Here's how the part is built. I have some questions about the finished solid (model axes, mm). A direction names the side the tool comes from. Round coordinates to 2 decimals unless told otherwise and drop trailing zeros. Order: outer loops, then holes, each group sorted by start corner. A loop starts at its lowest first (then second) coordinate and runs counter-clockwise, first axis right, second up. Notation, with made-up numbers: (26, 60.25) -> (57, 60.25) arc R14 ccw to (57, 67.25) -> close; hole circle Ø10 at (53, 67.25). An arc over 180 degrees is marked (long way). One line per item, written item: value.
```python
from build123d import *

# Parameters (mm, degrees)
F1_DEPTH = 15
F2_R     = 1.99999
F3_R     = 2
F4_R     = 1
F5_SIZE  = 1


# Not quite as in the source:
# - a fillet or chamfer is up to 0.001 mm smaller than in the source, because OpenCascade refuses the exact size


with BuildPart() as f1:
    # F0 (on Top) → F1 (new body)
    with BuildSketch(Plane.XY):
        with BuildLine():
            Line((2.5, -29.8956518578), (0, 0))
            Line((0, 0), (27, 0))
            Line((27, 0), (27, -30))
            ThreePointArc((27, -30), (45.6594117082, -45.2970585408), (57, -24))
            Line((57, -24), (52.5277389168, -24))
            ThreePointArc((52.5277389168, -24), (45.7143401039, -41.1741167757), (31, -30))
            Line((31, -30), (31, 4))
            Line((31, 4), (-4.348458452, 4))
            Line((-4.348458452, 4), (-1.4860869144, -30.2289851911))
            Line((-1.4860869144, -30.2289851911), (2.5, -29.8956518578))
        make_face()
    extrude(amount=F1_DEPTH)

    # F2 (radius 2 in the source; OpenCascade refuses exactly that, so slightly less here)
    f2_edges = [f1.edges().sort_by_distance(p)[0] for p in [
        (2.5, -29.895652, 7.5),
        (-1.486087, -30.228985, 7.5),
        (52.527739, -24, 7.5),
        (57, -24, 7.5),
    ]]
    fillet(f2_edges, radius=F2_R)

    # F3
    f3_edges = [f1.edges().sort_by_distance(p)[0] for p in [
        (31, 4, 7.5),
        (-4.348458, 4, 7.5),
    ]]
    fillet(f3_edges, radius=F3_R)

    # F4
    f4_edges = [f1.edges().sort_by_distance(p)[0] for p in [
        (0, 0, 7.5),
        (27, 0, 7.5),
    ]]
    fillet(f4_edges, radius=F4_R)

    # F5
    f5_edges = [f1.edges().sort_by_distance(p)[0] for p in [
        (1.211964, -14.492976, 15),
        (0.351135, -0.322997, 15),
        (1.867439, -29.360721, 15),
        (13.543557, 0, 15),
        (0.506957, -30.062319, 15),
        (26.707107, -0.292893, 15),
        (-0.951156, -29.596424, 15),
        (27, -15.5, 15),
        (-2.910013, -13.201309, 15),
        (44.919918, -45.426535, 15),
        (-3.646189, 3.354006, 15),
        (56.78664, -24.391198, 15),
        (13.412885, 4, 15),
        (55.598458, -24, 15),
        (30.414214, 3.414214, 15),
        (53.989656, -24.81182, 15),
        (31, -14, 15),
        (44.32507, -41.471013, 15),
        (1.211964, -14.492976, 0),
        (0.351135, -0.322997, 0),
        (1.867439, -29.360721, 0),
        (13.543557, 0, 0),
        (0.506957, -30.062319, 0),
        (26.707107, -0.292893, 0),
        (-0.951156, -29.596424, 0),
        (27, -15.5, 0),
        (-2.910013, -13.201309, 0),
        (44.919918, -45.426535, 0),
        (-3.646189, 3.354006, 0),
        (56.78664, -24.391198, 0),
        (13.412885, 4, 0),
        (55.598458, -24, 0),
        (30.414214, 3.414214, 0),
        (53.989656, -24.81182, 0),
        (31, -14, 0),
        (44.32507, -41.471013, 0),
    ]]
    chamfer(f5_edges, length=F5_SIZE)


solid = f1.part
```
Q1. For P1, Ø3, axis at x = 51, y = -27.5, coming from the -Z side; P2, Ø6.5, axis at y = -14.5, z = 6.5, coming from the +X side; P3, Ø3, axis at y = -15.5, z = 4, coming from the -X side; P4, Ø4, axis at x = 12.5, z = 8.5, coming from the -Y side, each with a flat end and sliding along its axis, tell me the tip position at first contact or that it passes through.
Answers:
P1: through
P2: x = 31
P3: x = -2.84
P4: y = 0
Q2. Which directions (+Z, -Z, +X, -X, +Y, -Y) give clear straight access to the entire face, cutting with the end or side of a thin tool? Please do faces 1 (the face through (26.966, -0.012, 0.618)), 2 (the face through (27, -15, 7)), 3 (the face through (0.06, -0.08, 0.62)).
Answers:
face 1: -Z, -Y
face 2: +Z, -Z, -Y
face 3: -Z
Q3. I want a section at A-A on y = -12.5. Write out the boundary of the cut face in (x, z).
Answers:
outline: (-2.97, 1) -> (-1.97, 0) -> (0.04, 0) -> (1.05, 1) -> (1.05, 14) -> (0.04, 15) -> (-1.97, 15) -> (-2.97, 14) -> close; (27, 1) -> (28, 0) -> (30, 0) -> (31, 1) -> (31, 14) -> (30, 15) -> (28, 15) -> (27, 14) -> close
Q4. I want a section at B-B on x = 42.6. Write out the boundary of the cut face in (y, z).
Answers:
outline: (-45.6, 1) -> (-44.6, 0) -> (-42.6, 0) -> (-41.6, 1) -> (-41.6, 14) -> (-42.6, 15) -> (-44.6, 15) -> (-45.6, 14) -> close
Q5. I need wall thicknesses on line 1 along X through (y, z) = (-29, 4); line 2 along Y through (x, z) = (42.6, 6.75); line 3 along Y through (x, z) = (6.5, 1.75). Which ranges of each line are inside material? Lowest first, please.
Answers:
line 1: -1.43 to 2.11, 27 to 31, 54.16 to 58.17
line 2: -45.6 to -41.6
line 3: 0 to 4
Q6. If we mould it in two halves opening along Y, with no side actions, what happens to faces 4 (the face through (31, -14, 7)), 5 (the face through (1.228, -14.681, 7.409)), 6 (the face through (30.4, 3.43, 7.59))? For each: pulls with the +Y half, pulls with the -Y half, needs draft (parallel to the pull), parting line crosses it, or undercut.
Answers:
face 4: needs draft
face 5: undercut
face 6: pulls with the +Y half
